Geometry check sheet. Reference: the model listing, model coordinates, mm. Face numbers are marked on the shaded views. A direction names the side the tool comes from. Give positions to 0.01 mm unless a question says otherwise; leave off trailing zeros. Order: outer loops, then holes, each group sorted by start corner. A loop starts at its lowest first (then second) coordinate and runs counter-clockwise, first axis right, second up. Notation, with made-up numbers: M 41.5,35.25 L 59.5,35.25 A13 ccw 59.5,43.25 Z; hole C 21,79 d4. An arc over 180 degrees is marked long. Use CSV: the item, a comma, the result in double quotes. Start each with the question number.
Autodesk Inventor part; units mm, degrees
ref_plane "YZ Plane" through (0, 0, 0) normal (1, 0, 0) x (0, 1, 0)
ref_plane "XZ Plane" through (0, 0, 0) normal (0, 1, 0) x (-1, 0, 0)
ref_plane "XY Plane" through (0, 0, 0) normal (0, 0, 1) x (1, 0, 0)
sketch "Sketch1" plane through (0, 0, 0) normal (0, 0, 1) x (1, 0, 0)
  line L0 (-20.4911, 10.9492) -> (11.2589, 10.9492)
  line L1 (11.2589, 10.9492) -> (11.2589, -20.8008)
  line L2 (11.2589, -20.8008) -> (-20.4911, -20.8008)
  line L3 (-20.4911, -20.8008) -> (-20.4911, 10.9492)
  point P0 (0, 0)
  dimension "d0" = 31.75
  dimension "d1" = 31.75
extrude "Extrusion1" add sketch "Sketch1" along normal blind 38.1
sketch "Sketch2" plane through (0, 0, 38.1) normal (0, 0, 1) x (1, 0, 0)
  line L0 (-20.4911, -20.8008) -> (11.2589, -20.8008)
  line L1 (11.2589, -20.8008) -> (-1.4411, 10.9492)
  line L2 (11.2589, 10.9492) -> (-20.4911, 10.9492)
  line L3 (-1.4411, 10.9492) -> (11.2589, 10.9492)
  line L4 (11.2589, -20.8008) -> (11.2589, 10.9492)
  line L5 (11.2589, 10.9492) -> (11.2589, -20.8008)
  point P0 (0, 0)
  dimension "d4" = 19.05
sketch "Sketch3" plane through (11.2589, -20.8008, 0) normal (1, 0, 0) x (0, 0, -1)
  line L0 (0, 31.75) -> (-38.1, 31.75)
  line L1 (0, 0) -> (-38.1, 0)
  line L2 (-25.4, 31.75) -> (-12.7, 31.75)
  line L3 (-12.7, 31.75) -> (-12.7, 0)
  line L4 (-12.7, 0) -> (-25.4, 0)
  line L5 (-25.4, 0) -> (-25.4, 31.75)
  line L6 (0, 31.75) -> (0, 0)
  line L7 (-38.1, 0) -> (-38.1, 31.75)
  point P0 (0, 20.8008)
  dimension "d5" = 12.7
  dimension "d6" = 12.7
extrude "Extrusion2" add sketch "Sketch3" along normal blind 25.4 contours L3 L1 L5 L0
sketch "Sketch4" plane through (11.2589, -20.8008, 25.4) normal (0, 0, 1) x (1, 0, 0)
  line L0 (0, 0) -> (25.4, 0)
  line L1 (25.4, 0) -> (15.2492, 31.75)
  line L2 (0, 31.75) -> (25.4, 31.75)
  line L3 (15.2492, 31.75) -> (25.4, 31.75)
  line L4 (25.4, 31.75) -> (25.4, 0)
  line L5 (25.4, 31.75) -> (25.4, 0)
  point P0 (-11.2589, 20.8008)
extrude "Extrusion3" cut sketch "Sketch4" against normal blind 25.4
extrude "Extrusion4" cut sketch "Sketch2" against normal blind 12.7
sketch "Sketch5" plane through (0, 0, 0) normal (0, 0, -1) x (-1, 0, 0)
  line L0 (-11.2589, 10.9492) -> (-11.2589, -20.8008)
  line L1 (-11.2589, -20.8008) -> (1.4411, 10.9492)
  line L2 (-11.2589, -20.8008) -> (1.4411, 10.9492)
  line L3 (20.4911, 10.9492) -> (-11.2589, 10.9492)
  line L4 (1.4411, 10.9492) -> (-11.2589, 10.9492)
  line L5 (-11.2589, 10.9492) -> (-11.2589, -20.8008)
  point P0 (0, 0)
extrude "Extrusion5" cut sketch "Sketch5" against normal blind 12.7
properties part number "Figure 7_28_1"
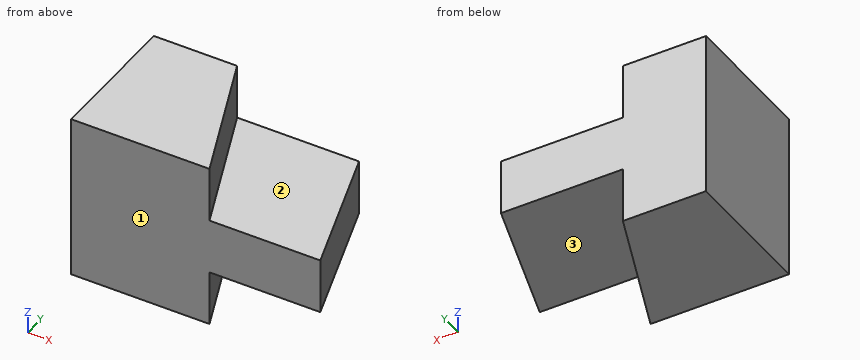
(1) Go/stop test with flat-tipped pins: P1, Ø6, axis at x = 14.5, y = -8, coming from the -Z side; P2, Ø3, axis at y = -4, z = 33.5, coming from the +X side; P3, Ø5, axis at x = 10, y = -3.5, coming from the +Z side. Record where each tip stops, or that it passes through.
(2) Access from +Z, -Z, +X, -X, +Y, -Y to the whole of each face (thin tool, end or side, straight path). Record for the marked faces 1, 2 and 3.
(3) Sectioned sample at B-B on y = 7.5. Record the cut outline in (x, z), then the cut area to 3 significant figures.
(4) Sectioned sample at D-D on x = 21. Record the cut outline in (y, z), then the cut area to 3 significant figures.
(5) Sectioned sample at A-A on x = 7.5. Record the cut outline in (y, z).
(6) Sectioned sample at C-C on z = 9. Record the cut outline in (x, y).
(7) Thickness scan on line 1 (Z direction, x = 10, y = 5.5); line 2 (X direction, y = -12, z = 24.5); line 3 (X direction, y = 5.5, z = 31). Record the ranges inside material, lowest first.
Responses:
1,P1,"z = 12.7"
1,P2,"x = 5.14"
1,P3,"z = 25.4"
2,face 1,"+Z, -Z, +X, -X, -Y"
2,face 2,"+Z, +X, +Y"
2,face 3,"-Z, +X, +Y"
3,outline,"M -20.49,0 L -0.06,0 L -0.06,12.7 L 27.61,12.7 L 27.61,25.4 L -0.06,25.4 L -0.06,38.1 L -20.49,38.1 Z"
3,area,"1,130 mm2"
4,outline,"M -20.8,12.7 L 10.95,12.7 L 10.95,25.4 L -20.8,25.4 Z"
4,area,"403 mm2"
5,outline,"M -20.8,0 L -11.4,0 L -11.4,12.7 L 10.95,12.7 L 10.95,25.4 L -11.4,25.4 L -11.4,38.1 L -20.8,38.1 Z"
6,outline,"M -20.49,-20.8 L 11.26,-20.8 L -1.44,10.95 L -20.49,10.95 Z"
7,line 1,"12.7 to 25.4"
7,line 2,"-20.49 to 33.85"
7,line 3,"-20.49 to 0.74"
